Read the model definition and answer for the solid it produces. Units are mm, in the model's axes. Coordinates: 2 decimals unless noted, no trailing zeros. Loops run counter-clockwise (first coordinate to the right, second up) from the corner with the lowest first, then second, coordinate; pieces in that order, holes last. Notation, with made-up numbers: M 14,4 L 51,4 A14 ccw 51,18 Z; hole C 3,76 d10. An arc over 180 degrees is marked long. Use one line per item in the form item = value. Start each with the question number.
1. The part is cut by section B-B (x = 29.5). Give the vertices of the cut face in (y, z), plus the area to 3 significant figures.
2. The part is cut by section A-A (z = 0.65). Give the vertices of the cut face in (x, y).
3. The part is cut by section C-C (y = 28.5). Give the vertices of the cut face in (x, z).
4. Find the intervals of material crossed by probe 1 along X at (y, z) = (39.5, -1); probe 2 along Y at (x, z) = (-17.5, -0.8), in increasing order. Write a range as [from, to].
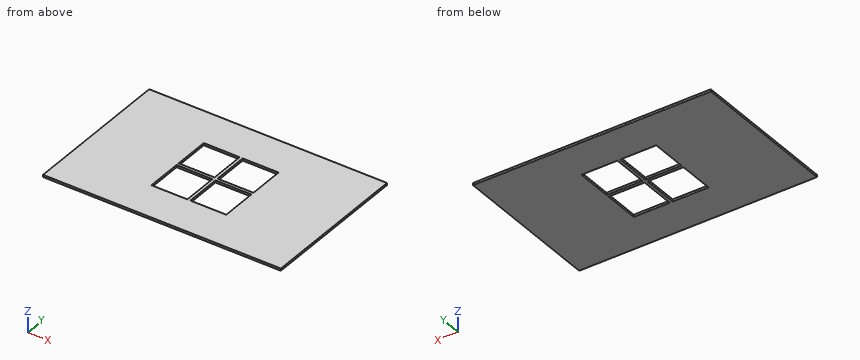
Autodesk Inventor part; units mm, degrees
ref_plane "YZ Plane" through (0, 0, 0) normal (1, 0, 0) x (0, 1, 0)
ref_plane "XZ Plane" through (0, 0, 0) normal (0, 1, 0) x (-1, 0, 0)
ref_plane "XY Plane" through (0, 0, 0) normal (0, 0, 1) x (1, 0, 0)
sketch "Szkic1" plane through (0, 0, 0) normal (0, 0, 1) x (1, 0, 0)
  line L0 (-159, 101.5) -> (159, 101.5)
  line L1 (159, 101.5) -> (159, -101.5)
  line L2 (159, -101.5) -> (-159, -101.5)
  line L3 (-159, -101.5) -> (-159, 101.5)
  line L4 (-159, 101.5) -> (159, -101.5) construction
  line L5 (159, 101.5) -> (-159, -101.5) construction
  point P0 (0, 0)
  dimension "d0" = 318
  dimension "d1" = 203
extrude "Wyciągnięcie proste1" add sketch "Szkic1" along normal mid plane 3
sketch "Szkic2" plane through (0, 0, 1.5) normal (0, 0, 1) x (1, 0, 0)
  line L0 (50, -50) -> (-50, -50)
  line L1 (-50, -50) -> (-50, 50)
  line L2 (-50, 50) -> (50, 50)
  line L3 (50, 50) -> (50, -50)
  line L4 (50, -50) -> (-50, 50) construction
  line L5 (-50, -50) -> (50, 50) construction
  line L6 (-2, 50) -> (2, 50)
  line L7 (2, 50) -> (2, -50)
  line L8 (2, -50) -> (-2, -50)
  line L9 (-2, -50) -> (-2, 50)
  line L10 (-50, 2) -> (50, 2)
  line L11 (50, 2) -> (50, -2)
  line L12 (50, -2) -> (-50, -2)
  line L13 (-50, -2) -> (-50, 2)
  line L14 (159, -101.5) -> (159, 101.5)
  line L15 (159, 101.5) -> (-159, 101.5)
  point P0 (0, 0)
  point P1 (2, -2)
  point P2 (-2, -2)
  point P3 (-50, -2)
  point P4 (-2, -50)
  point P5 (2, 2)
  point P6 (50, 2)
  point P7 (2, 50)
  point P8 (-2, 2)
  dimension "d4" = 100
  dimension "d5" = 100
  dimension "d6" = 4
  dimension "d7" = 100
  dimension "d8" = 48
  dimension "d9" = 4
  dimension "d10" = 48
extrude "Wyciągnięcie proste2" cut sketch "Szkic2" against normal through all contours L0 L7 L12 L3 | L0 L1 L12 L9 | L10 L7 L2 L3 | L10 L1 L2 L9
properties part number "LeftWall_Window"
Computed values:
q1.outline = M -101.5,-1.5 L -50,-1.5 L -50,1.5 L -101.5,1.5 Z; M -2,-1.5 L 2,-1.5 L 2,1.5 L -2,1.5 Z; M 50,-1.5 L 101.5,-1.5 L 101.5,1.5 L 50,1.5 Z
q1.area = 321 mm²
q2.outline = M -159,-101.5 L 159,-101.5 L 159,101.5 L -159,101.5 Z; hole M -50,-50 L -2,-50 L -2,-2 L -50,-2 Z; hole M -50,2 L -2,2 L -2,50 L -50,50 Z; hole M 2,-50 L 50,-50 L 50,-2 L 2,-2 Z; hole M 2,2 L 50,2 L 50,50 L 2,50 Z
q3.outline = M -159,-1.5 L -50,-1.5 L -50,1.5 L -159,1.5 Z; M -2,-1.5 L 2,-1.5 L 2,1.5 L -2,1.5 Z; M 50,-1.5 L 159,-1.5 L 159,1.5 L 50,1.5 Z
q4.probe_1 = [-159, -50], [-2, 2], [50, 159]
q4.probe_2 = [-101.5, -50], [-2, 2], [50, 101.5]
